Could you check a few things on this drawing? It's one solid part, dimensions in mm from its lowest x, y, z. Round coordinates to 2 decimals unless told otherwise and drop trailing zeros. Loops run counter-clockwise (first coordinate to the right, second up) from the corner with the lowest first, then second, coordinate; pieces in that order, holes last. Notation, with made-up numbers: (59.5, 36) -> (68.5, 36) arc R28 ccw to (68.5, 67) -> close; hole circle Ø3 at (-39.75, 61.25). An arc over 180 degrees is marked (long way). Write each question's results on one line, items separated by ' | '.
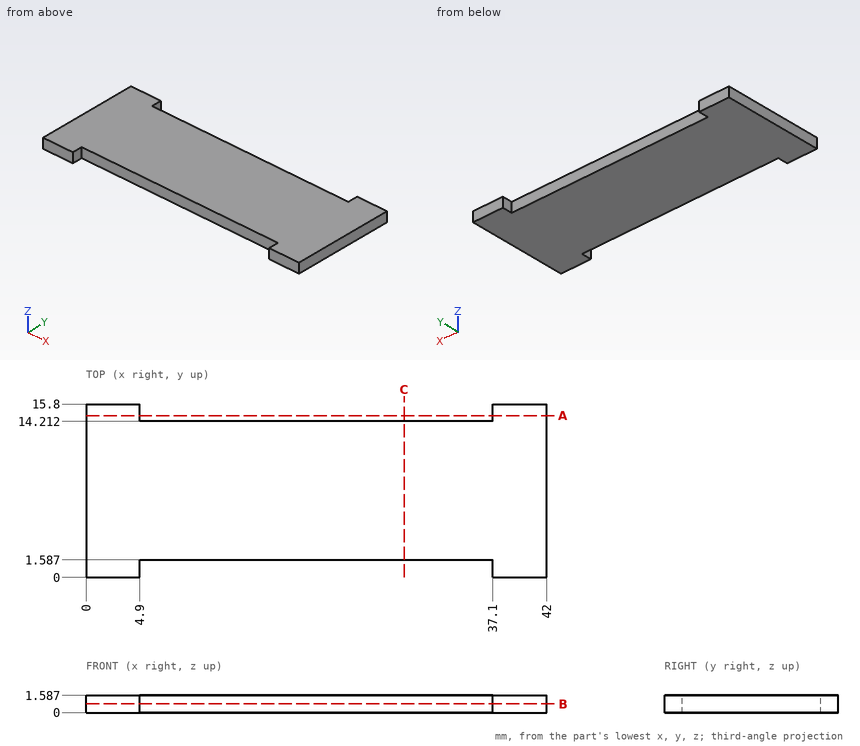
1) I want a section at A-A, the plane y = 14.75. Write out the boundary of the cut face in (x, z).
Model answer:
outline: (0, 0) -> (4.9, 0) -> (4.9, 1.59) -> (0, 1.59) -> close; (37.1, 0) -> (42, 0) -> (42, 1.59) -> (37.1, 1.59) -> close
2) I want a section at C-C, the plane x = 29. Write out the boundary of the cut face in (y, z).
Model answer:
outline: (1.59, 0) -> (14.21, 0) -> (14.21, 1.59) -> (1.59, 1.59) -> close
3) I need wall thicknesses on line 1 (Y direction, x = 17.5, z = 1.2). Which ranges of the line are inside material? Lowest first, please.
Model answer:
line 1: y = 1.59 to 14.21
4) I'm going to push flat-ended pins straight in: pin 1 (0.5 mm diameter, centred on x = 16, z = 0.5, fed in from +Y); pin 2 (0.8 mm diameter, centred on x = 16.5, z = 0.5, fed in from -Y). Where does each tip first touch, or does it pass through?
Model answer:
pin 1: stops at y = 14.21 | pin 2: stops at y = 1.59
5) I want a section at B-B, the plane z = 0.8. Write out the boundary of the cut face in (x, y), plus the area to 3 significant figures.
Model answer:
outline: (0, 0) -> (4.9, 0) -> (4.9, 1.59) -> (37.1, 1.59) -> (37.1, 0) -> (42, 0) -> (42, 15.8) -> (37.1, 15.8) -> (37.1, 14.21) -> (4.9, 14.21) -> (4.9, 15.8) -> (0, 15.8) -> close | area: 561 mm2
